```python
from build123d import *

# Parameters (mm, degrees)
F1_DEPTH = 60
F2_W     = 20
F2_H     = 15
F3_DEPTH = 50
F5_DEPTH = 60.001
F6_W     = 10
F6_H     = 20
F7_DEPTH = 30.001
F8_DEPTH = 15.0010001


with BuildPart() as f1:
    # F0 (on Front) → F1 (new body)
    with BuildSketch(Plane.XZ):
        with BuildLine():
            ThreePointArc((0, 25), (-17.6776695297, 17.6776695297), (-25, 0))
            Line((-25, 0), (0, 0))
            Line((0, 0), (0, 25))
        make_face()
        with BuildLine():
            ThreePointArc((0, 30), (-21.2132034356, 21.2132034356), (-30, 0))
            Line((-30, 0), (-25, 0))
            ThreePointArc((-25, 0), (-17.6776695297, 17.6776695297), (0, 25))
            Line((0, 25), (0, 30))
        make_face()
    extrude(amount=-F1_DEPTH)

    # F2 (on face) → F3 (join)
    with BuildSketch(Plane.YZ):
        with Locations((50, 7.5)):
            Rectangle(F2_W, F2_H)
    extrude(amount=-F3_DEPTH)

    # F0 (on Front) → F5 (cut, through all)
    with BuildSketch(Plane.XZ):
        with BuildLine():
            ThreePointArc((0, 25), (-17.6776695297, 17.6776695297), (-25, 0))
            Line((-25, 0), (0, 0))
            Line((0, 0), (0, 25))
        make_face()
    extrude(amount=-F5_DEPTH, mode=Mode.SUBTRACT)

    # F6 (on Top) → F7 (cut, through all)
    with BuildSketch(Plane.XY):
        with Locations((-5, 10)):
            Rectangle(F6_W, F6_H)
        with BuildLine():
            Line((-10, 20), (0, 20))
            Line((0, 20), (0, 30))
            ThreePointArc((0, 30), (-7.0710678119, 27.0710678119), (-10, 20))
        make_face()
    extrude(amount=F7_DEPTH, mode=Mode.SUBTRACT)

    # F4 (on face) → F8 (cut, through all)
    with BuildSketch(Plane.XY.offset(15)):
        with BuildLine():
            ThreePointArc((-40, 40), (-47.0710678119, 42.9289321881), (-50, 50))
            Line((-50, 50), (-50, 40))
            Line((-50, 40), (-40, 40))
        make_face()
        with BuildLine():
            Line((-40, 60), (-50, 60))
            Line((-50, 60), (-50, 50))
            ThreePointArc((-50, 50), (-47.0710678119, 57.0710678119), (-40, 60))
        make_face()
        with BuildLine():
            Line((-40, 50), (-45, 50))
            ThreePointArc((-45, 50), (-43.5355339059, 46.4644660941), (-40, 45))
            Line((-40, 45), (-40, 50))
        make_face()
        with BuildLine():
            Line((-35, 50), (-40, 50))
            Line((-40, 50), (-40, 45))
            ThreePointArc((-40, 45), (-36.4644660941, 46.4644660941), (-35, 50))
        make_face()
        with BuildLine():
            ThreePointArc((-35, 50), (-36.4644660941, 53.5355339059), (-40, 55))
            Line((-40, 55), (-40, 50))
            Line((-40, 50), (-35, 50))
        make_face()
        with BuildLine():
            ThreePointArc((-40, 55), (-43.5355339059, 53.5355339059), (-45, 50))
            Line((-45, 50), (-40, 50))
            Line((-40, 50), (-40, 55))
        make_face()
    extrude(amount=-F8_DEPTH, mode=Mode.SUBTRACT)

    # F9: F1 across plane


with BuildPart() as f1_1:
    add(f1.part)
    add(f1.part.mirror(Plane.YZ))


solid = f1_1.part
```
Verification items for the finished model (mm, model axes). A direction names the side the tool comes from. Coordinates: 2 decimals unless noted, no trailing zeros. Order: outer loops, then holes, each group sorted by start corner. A loop starts at its lowest first (then second) coordinate and runs counter-clockwise, first axis right, second up. Notation, with made-up numbers: (30.5, 15.5) - (36.5, 15.5) arc R26 cw to (36.5, 45.5) - close; hole circle Ø6 at (45.25, 53). An arc over 180 degrees is marked (long way). Return JSON: item names as keys, results as strings.
(1) Section check C-C, the plane y = 36.5. Record the cut outline in (x, z), and give its area (3 significant figures).
Filled sheet:
{"outline": "(-30, 0) - (-25, 0) arc R25 cw to (25, 0) - (30, 0) arc R30 ccw to start", "area": "432 mm^2"}
(2) Section check A-A, the plane y = 14.5. Record the cut outline in (x, z), and give its area (3 significant figures).
Filled sheet:
{"outline": "(-30, 0) - (-25, 0) arc R25 cw to (-10, 22.91) - (-10, 28.28) arc R30 ccw to start; (10, 22.91) arc R25 cw to (25, 0) - (30, 0) arc R30 ccw to (10, 28.28) - close", "area": "330 mm^2"}
(3) Section check B-B, the plane z = 7.5. Record the cut outline in (x, y), and give its area (3 significant figures).
Filled sheet:
{"outline": "(-40, 40) - (-29.05, 40) - (-29.05, 0) - (-23.85, 0) - (-23.85, 60) - (-40, 60) arc R10 ccw to start; (23.85, 0) - (29.05, 0) - (29.05, 40) - (40, 40) arc R10 ccw to (40, 60) - (23.85, 60) - close; hole circle Ø10 at (-40, 50); hole circle Ø10 at (40, 50)", "area": "1,220 mm^2"}
(4) Mould release check, pull along X, two halves, no side actions. Record for faces 5 (the cylindrical face through (9.64, 29.58, 28.41)), 6 (the flat face through (-35, 48, 15)), 7 (the flat face through (10, 10, 26)): pulls with the +X half, pulls with the -X half, needs draft (parallel to the pull), parting line crosses it, or undercut.
Filled sheet:
{"face 5": "parting line crosses it", "face 6": "needs draft", "face 7": "undercut"}
(5) Section check D-D, the plane x = -44. Record the cut outline in (y, z), and give its area (3 significant figures).
Filled sheet:
{"outline": "(40.83, 0) - (47, 0) - (47, 15) - (40.83, 15) - close; (53, 0) - (59.17, 0) - (59.17, 15) - (53, 15) - close", "area": "185 mm^2"}
(6) Thickness scan on line 1 along X through (y, z) = (48.5, 4); line 2 along X through (y, z) = (46.5, 6); line 3 along X through (y, z) = (29.5, 13). Record the ranges inside material, lowest first.
Filled sheet:
{"line 1": "x = -49.89 to -44.77, -35.23 to -24.68, 24.68 to 35.23, 44.77 to 49.89", "line 2": "x = -49.37 to -43.57, -36.43 to -24.27, 24.27 to 36.43, 43.57 to 49.37", "line 3": "x = -27.04 to -21.35, 21.35 to 27.04"}
(7) Access from +Z, -Z, +X, -X, +Y, -Y to the whole of each face (thin tool, end or side, straight path). Record for faces 1 (the flat face through (-34, 40, 7)), 2 (the flat face through (34, 40, 7)), 3 (the flat face through (35, 48, 15)), 4 (the flat face through (-10, 10, 26)).
Filled sheet:
{"face 1": "+Z, -X, -Y", "face 2": "+Z, +X, -Y", "face 3": "+Z, +X, +Y, -Y", "face 4": "+Z, -Z, -Y"}
(8) Go/stop test with flat-tipped pins: pin 1 (11 mm diameter, centred on x = -33, z = 11, fed in from -Y); pin 2 (3 mm diameter, centred on x = -10.5, y = 29.5, fed in from +Z); pin 3 (2.5 mm diameter, centred on y = 15, z = 27, fed in from -X); pin 4 (4 mm diameter, centred on x = 30.5, z = 10, fed in from -Y). Record where each tip stops, or that it passes through.
Filled sheet:
{"pin 1": "stops at y = 0", "pin 2": "stops at z = 28.62", "pin 3": "stops at x = -15.39", "pin 4": "stops at y = 40"}
